Here's how the part is built. I have some questions about the finished solid (model axes, mm). A direction names the side the tool comes from. Give positions to 0.01 mm unless a question says otherwise; leave off trailing zeros. Write each loop counter-clockwise with the first axis right and the second up, starting at its lowest first coordinate (ties: lowest second). Pieces come first, ordered by that corner, then holes. Notation, with made-up numbers: (56.25, -27.5) -> (73.25, -27.5) arc R12 ccw to (73.25, -19.5) -> close; hole circle Ø9 at (-7.5, 7). An arc over 180 degrees is marked (long way). Use one line per item in the form item = value.
Autodesk Inventor part; units mm, degrees
ref_plane "YZ Plane" through (0, 0, 0) normal (1, 0, 0) x (0, 1, 0)
ref_plane "XZ Plane" through (0, 0, 0) normal (0, 1, 0) x (-1, 0, 0)
ref_plane "XY Plane" through (0, 0, 0) normal (0, 0, 1) x (1, 0, 0)
sketch "Sketch1" plane through (0, 0, 0) normal (0, 0, 1) x (1, 0, 0)
  line L0 (13, 0) -> (13, 7)
  line L1 (0, 7) -> (0, 0)
  arc A0 (13, 7) -> (0, 7) centre (6.5, 7) ccw
  line L2 (10, 0) -> (10, -5.5)
  line L3 (10, -5.5) -> (3, -5.5)
  line L4 (3, -5.5) -> (3, 0)
  line L5 (0, 0) -> (3, 0)
  line L6 (10, 0) -> (13, 0)
  circle A1 centre (6.5, 7) radius 1.5
  dimension "d0" = 7
  dimension "d1" = 3
  dimension "d2" = 3
  dimension "d3" = 7
  dimension "d7" = 3
  dimension "d10" = 5.5
  dimension "d11" = 7
extrude "Extrusion2" add sketch "Sketch1" along normal blind 3
properties part number "Gripper V 6.0 base tab 3mm"
Q1. I want a section at A-A, the plane x = 6.5. Write out the boundary of the cut face in (y, z), and give its area (3 significant figures).
Result set:
outline = (-5.5, 0) -> (5.5, 0) -> (5.5, 3) -> (-5.5, 3) -> close; (8.5, 0) -> (13.5, 0) -> (13.5, 3) -> (8.5, 3) -> close
area = 48.0 mm2
Q2. I want a section at C-C, the plane x = 9.25. Write out the boundary of the cut face in (y, z).
Result set:
outline = (-5.5, 0) -> (12.89, 0) -> (12.89, 3) -> (-5.5, 3) -> close
Q3. I want a section at D-D, the plane y = 9. Write out the boundary of the cut face in (x, z), and give its area (3 significant figures).
Result set:
outline = (0.32, 0) -> (12.68, 0) -> (12.68, 3) -> (0.32, 3) -> close
area = 37.1 mm2
Q4. Which directions (+Z, -Z, +X, -X, +Y, -Y) give clear straight access to the entire face, cutting with the end or side of a thin tool? Please do faces 4 (the face through (1, 0, 1)), 5 (the face through (10, -3, 1)), 6 (the face through (6.4, 13.5, 1.5)).
Result set:
face_4 = +Z, -Z, -X, -Y
face_5 = +Z, -Z, +X, -Y
face_6 = +Z, -Z, +Y
Q5. If I drill on line 1 along Y through (x, z) = (6.5, 0.8); line 2 along X through (y, z) = (-0.75, 2.2); line 3 along X through (y, z) = (6, 1), over which ranges is the centre line in solid material (lowest first)? Write a range as from..to.
Result set:
line_1 = -5.5..5.5, 8.5..13.5
line_2 = 3..10
line_3 = 0..5.38, 7.62..13
Q6. Will these pins go through, and if not, where does the flat tip stop? pin 1 Ø1.5 at (y, z) = (0, 1) entering from -X; pin 2 Ø1.5 at (x, z) = (1.5, 1.5) entering from -Y; pin 3 Ø0.9 at (y, z) = (-2.5, 2) entering from -X.
Result set:
pin_1 = 0
pin_2 = 0
pin_3 = 3
Q7. I want a section at B-B, the plane z = 0.45. Write out the boundary of the cut face in (x, y).
Result set:
outline = (0, 0) -> (3, 0) -> (3, -5.5) -> (10, -5.5) -> (10, 0) -> (13, 0) -> (13, 7) arc R6.5 ccw to (0, 7) -> close; hole circle Ø3 at (6.5, 7)
Q8. If we mould it in two halves opening along X, with no side actions, what happens to faces 1 (the face through (5.3, 7.9, 1.5)), 2 (the face through (6, 4, 0)), 3 (the face through (0, 4, 1))? For each: +X half, -X half, draft (parallel to the pull), parting line (faces both ways), or undercut.
Result set:
face_1 = undercut
face_2 = draft
face_3 = -X half
